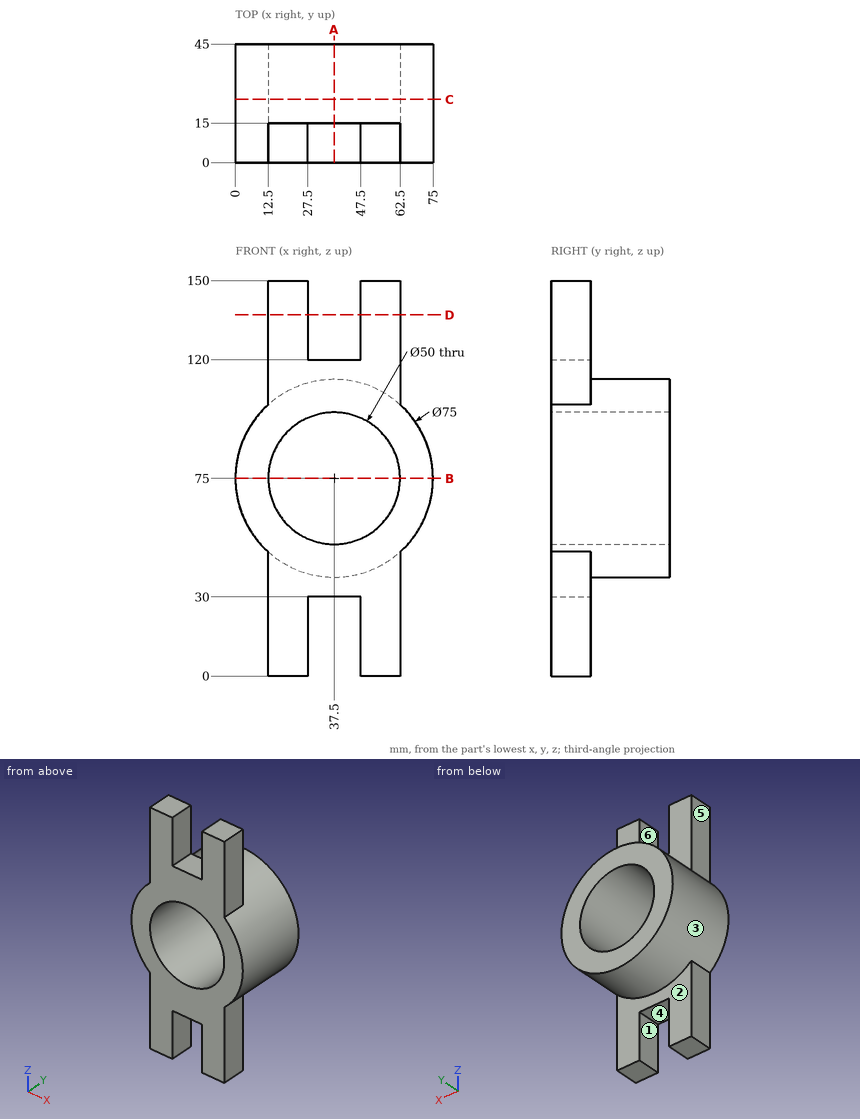
The drawing under review shows one solid part. Ordinate dimensions are in mm from its lowest x, y, z. A direction names the side the tool comes from. Round coordinates to 2 decimals unless told otherwise and drop trailing zeros. Write each loop counter-clockwise with the first axis right and the second up, starting at its lowest first coordinate (ties: lowest second). Pieces come first, ordered by that corner, then holes. Notation, with made-up numbers: (0.25, -11.5) - (6.25, -11.5) arc R29 ccw to (6.25, 14.5) - close; hole circle Ø10 at (50.25, 4). An arc over 180 degrees is marked (long way). Put each result on its own line as item: value.
Q1. We need section D-D (z = 137). Give the boundary of the cut face in (x, y), and give its area (3 significant figures).
Solved:
outline: (12.5, 0) - (27.5, 0) - (27.5, 15) - (12.5, 15) - close; (47.5, 0) - (62.5, 0) - (62.5, 15) - (47.5, 15) - close
area: 450 mm2
Q2. We need section C-C (y = 24). Give the boundary of the cut face in (x, z), and give its area (3 significant figures).
Solved:
outline: circle Ø75 at (37.5, 75); hole circle Ø50 at (37.5, 75)
area: 2,450 mm2
Q3. Machinability: for the marked faces 4, 5 and 6, which of the approach directions +Z, -Z, +X, -X, +Y, -Y give a long, thin tool a straight path to every point of the face, cutting with its end or side? Answer none if there is none.
Solved:
face 4: -Z, +Y, -Y
face 5: +Z, -X, +Y, -Y
face 6: +Z, +Y, -Y
Q4. We need section A-A (x = 37.5). Give the boundary of the cut face in (y, z).
Solved:
outline: (0, 30) - (15, 30) - (15, 37.5) - (45, 37.5) - (45, 50) - (0, 50) - close; (0, 100) - (45, 100) - (45, 112.5) - (15, 112.5) - (15, 120) - (0, 120) - close
Q5. Mouldability with a two-part tool opening along X and no side actions: class the marked faces 1, 2 and 3 as released by +X, released by -X, zero draft, split by the parting line, or undercut.
Solved:
face 1: undercut
face 2: zero draft
face 3: split by the parting line
Q6. Wall thickness on probe 1 along X at (y, z) = (24, 75); probe 2 along Z at (x, y) = (37, 11) (3 decimals); probe 3 along Z at (x, y) = (31.5, 2.5): over which ranges is each line inside the solid? List them lowest first.
Solved:
probe 1: x = 0 to 12.5, 62.5 to 75
probe 2: z = 30 to 50.005, 99.995 to 120
probe 3: z = 30 to 50.73, 99.27 to 120
Q7. We need section B-B (z = 75). Give the boundary of the cut face in (x, y).
Solved:
outline: (0, 0) - (12.5, 0) - (12.5, 45) - (0, 45) - close; (62.5, 0) - (75, 0) - (75, 45) - (62.5, 45) - close
Q8. Insertion check: pin 1 Ø6 at (y, z) = (15, 90.5) entering from -X; pin 2 Ø12 at (y, z) = (10.5, 11.5) entering from +X; pin 3 Ø7.5 at (y, z) = (7.5, 137.5) entering from -X. Each pin has a flat end and moves straight along its axis. Give the tip position at first contact, or say it passes through.
Solved:
pin 1: stops at x = 2.14
pin 2: stops at x = 62.5
pin 3: stops at x = 12.5
